Check sheet for the modelled part. Datum: model origin and axes. Units: mm. A direction names the side the tool comes from. Round coordinates to 2 decimals unless told otherwise and drop trailing zeros. Order: outer loops, then holes, each group sorted by start corner. A loop starts at its lowest first (then second) coordinate and runs counter-clockwise, first axis right, second up.
```python
from build123d import *

# Parameters (mm, degrees)
SKETCH1_R           = 16
BOSS_EXTRUDE1_DEPTH = 40
RIB1_REACH          = 99.617
SKETCH5_WALL_W      = 273.54941501
SKETCH5_WALL_H      = 10
SKETCH8_W           = 20
SKETCH8_H           = 8
CUT_EXTRUDE2_DEPTH  = 40


with BuildPart() as part:
    # Sketch1 → Boss-Extrude1 (new body)
    with BuildSketch(Plane.XY):
        with BuildLine():
            Line((-44.962686567, 12), (-44.962686567, 44))
            ThreePointArc((-44.962686567, 44), (-18.962686567, 70), (7.037313433, 44))
            Line((7.037313433, 44), (7.037313433, 12))
            Line((7.037313433, 12), (55.037313433, 12))
            Line((55.037313433, 12), (55.037313433, 0))
            Line((55.037313433, 0), (-44.962686567, 0))
            Line((-44.962686567, 0), (-44.962686567, 12))
        make_face()
        with Locations((-18.962686567, 44)):
            Circle(SKETCH1_R, mode=Mode.SUBTRACT)
    extrude(amount=-BOSS_EXTRUDE1_DEPTH)

    # Sketch5 wall → Rib1 (add, up to next)
    with BuildSketch(Plane(origin=(26.769481976, 37.630640297, -40), x_dir=(-0.740818472674, 0.671705285483, 0), z_dir=(-0.671705285483, -0.740818472674, 0)), mode=Mode.PRIVATE) as rib1_sk1:
        with Locations((0, -5)):
            Rectangle(SKETCH5_WALL_W, SKETCH5_WALL_H)
    rib1_tool1 = extrude(rib1_sk1.sketch, amount=RIB1_REACH, mode=Mode.PRIVATE) - part.part
    add(rib1_tool1.solids().sort_by_distance((26.769481976, 37.630640297, -40))[0])

    # Sketch8 → Cut-Extrude2 (cut)
    with BuildSketch(Plane(origin=(0, 12, 0), x_dir=(1, 0, 0), z_dir=(0, 1, 0))):
        with Locations((37.559585663, 14)):
            Rectangle(SKETCH8_W, SKETCH8_H)
    extrude(amount=-CUT_EXTRUDE2_DEPTH, mode=Mode.SUBTRACT)


solid = part.part
```
Item 1: Scan lines: line 1 along X through (y, z) = (8.5, -11); line 2 along Y through (x, z) = (20, -13); line 3 along Z through (x, y) = (39.5, 6.5). Record each from-to range of solid material in increasing order.
Answer:
line 1: x = -44.96 to 27.56, 47.56 to 55.04
line 2: y = 0 to 12
line 3: z = -40 to -18, -10 to 0
Item 2: Release check for a two-part mould opening along Z. For faces 1 (the flat face through (1, 22, -40)), 2 (the flat face through (27.56, 6, -14)), 3 (the cylindrical face through (-21.046, 59.864, -19.72)) record: released by +Z, released by -Z, zero draft, split by the parting line, or undercut.
Answer:
face 1: released by -Z
face 2: undercut
face 3: zero draft
Item 3: Sectioned sample at D-D (y = 18.5). Record the cut outline in (x, z).
Answer:
outline: (-44.96, -40) - (47.87, -40) - (47.87, -30) - (7.04, -30) - (7.04, 0) - (-44.96, 0) - close
Item 4: Sectioned sample at B-B (z = -4). Record the cut outline in (x, y).
Answer:
outline: (-44.96, 0) - (55.04, 0) - (55.04, 12) - (7.04, 12) - (7.04, 44) arc R26 ccw to (-44.96, 44) - close; hole circle Ø32 at (-18.96, 44)
Item 5: Sectioned sample at A-A (z = -15.5). Record the cut outline in (x, y), and give its area (3 significant figures).
Answer:
outline: (-44.96, 0) - (27.56, 0) - (27.56, 12) - (7.04, 12) - (7.04, 44) arc R26 ccw to (-44.96, 44) - close; (47.56, 0) - (55.04, 0) - (55.04, 12) - (47.56, 12) - close; hole circle Ø32 at (-18.96, 44)
area: 2,880 mm2
Item 6: Go/stop test with flat-tipped pins: P1, Ø5, axis at y = 51.5, z = -31, coming from the +X side; P2, Ø15, axis at y = 28.5, z = -12.5, coming from the +X side; P3, Ø4, axis at x = 28.5, z = -22.5, coming from the +Y side. Record where each tip stops, or that it passes through.
Answer:
P1: stops at x = 14.23
P2: stops at x = 7.04
P3: stops at y = 12
Item 7: Access from +Z, -Z, +X, -X, +Y, -Y to the whole of each face (thin tool, end or side, straight path). Record for faces 4 (the flat face through (27.17, 37.27, -35.07)), 5 (the flat face through (21, 31, -30)), 6 (the flat face through (37, 6, -10)), 7 (the cylindrical face through (-19.534, 69.994, -19.72)).
Answer:
face 4: +Z, -Z, +X, +Y
face 5: +Z, +X, +Y
face 6: +Y, -Y
face 7: +Z, +Y
Item 8: Sectioned sample at C-C (x = -30). Record the cut outline in (y, z), and give its area (3 significant figures).
Answer:
outline: (0, -40) - (32.42, -40) - (32.42, 0) - (0, 0) - close; (55.58, -40) - (67.54, -40) - (67.54, 0) - (55.58, 0) - close
area: 1,770 mm2
